Job drawing, mm, ordinate dimensions from the low corner. One solid piece. A direction names the side the tool comes from. Give positions to 0.01 mm unless a question says otherwise; leave off trailing zeros. Order: outer loops, then holes, each group sorted by start corner. A loop starts at its lowest first (then second) coordinate and runs counter-clockwise, first axis right, second up.
1. Which spindle directions (+Z, -Z, +X, -X, +Y, -Y) get a long thin tool onto all of the face, cutting with end or side? Do the marked faces 4 and 5. Say none if no direction does.
2. Drop flat-ended pins along their axis: pin 1 Ø1.5 at (y, z) = (101.5, 3) entering from +X; pin 2 Ø4 at (y, z) = (43.5, 5) entering from +X; pin 3 Ø2 at (x, y) = (3, 80) entering from +Z. Give the stop position or say it passes through.
3. Probe line 1 (Y direction, x = 7.75, z = 9); line 2 (Y direction, x = 12.5, z = 9); line 3 (Y direction, x = 9.5, z = 12.75). List the from-to ranges inside material, lowest first.
4. Mould opens along Y. For the marked faces 1, 2 and 3 say: +Y half, -Y half, draft (parallel to the pull), parting line (faces both ways), or undercut.
5. Slice it at B-B on y = 51. List the corners of the cut face in (x, z), and give its area (3 significant figures).
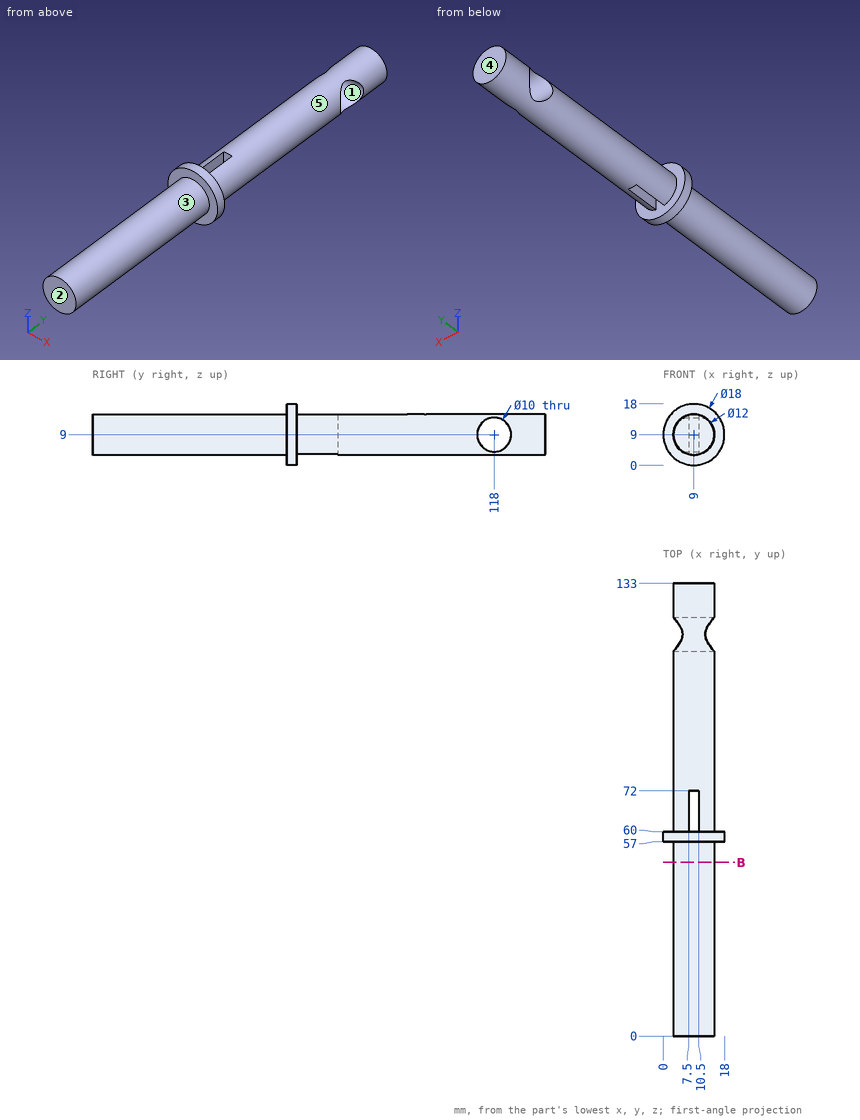
Data:
1. face 4: +Z, -Z, +X, -X, +Y
1. face 5: +Y
2. pin 1: stops at x = 11.9
2. pin 2: stops at x = 14.66
2. pin 3: stops at z = 12.32
3. line 1: y = 0 to 60, 72 to 113, 123 to 133
3. line 2: y = 0 to 113, 123 to 133
3. line 3: y = 0 to 60, 72 to 114.69, 121.31 to 133
4. face 1: undercut
4. face 2: -Y half
4. face 3: draft
5. outline: circle Ø12 at (9, 9)
5. area: 113 mm2
